Input: part model. Units: mm. Frame: model coordinates. A direction names the side the tool comes from. Give positions to 0.01 mm unless a question says otherwise; leave off trailing zeros. Loops run counter-clockwise (first coordinate to the right, second up) from the corner with the lowest first, then second, coordinate; pieces in that order, holes last. Notation, with made-up numbers: (66, 61) -> (95, 61) arc R22 cw to (95, 82) -> close; hole circle Ø8 at (-23.5, 61). An arc over 180 degrees is marked (long way). Use CSV: the item, a comma, the result in double quotes.
```python
from build123d import *

# Parameters (mm, degrees)
FILLET1_R = 3
FILLET2_R = 3


with BuildPart() as part:
    # Sketch2 → Revolve1 (revolve)
    with BuildSketch(Plane(origin=(0, 0, 0), x_dir=(0, 0, -1), z_dir=(1, 0, 0))):
        Polygon((0, 0), (0, 100), (33.5, 100), (33.5, 27), (31.5, 27), (31.5, 25), (33.5, 25), (33.5, 0), align=None)
    revolve(axis=Axis((0, 0, 0), (0, 1, 0)))

    # Fillet1
    fillet1_edges = [part.edges().sort_by_distance(p)[0] for p in [
        (0, 100, 33.5),
    ]]
    fillet(fillet1_edges, radius=FILLET1_R)

    # Fillet2
    fillet2_edges = [part.edges().sort_by_distance(p)[0] for p in [
        (0, 0, 33.5),
    ]]
    fillet(fillet2_edges, radius=FILLET2_R)


solid = part.part
```
1) Reachability of faces 4 (the cylindrical face through (32.703, 13.846, 7.262)), 5 (the flat face through (20, 25, 25)) from +Z, -Z, +X, -X, +Y, -Y: full face, straight path, thin tool, end or side. Return the list, or none.
From the geometry:
face 4,"+Y, -Y"
face 5,"none"
2) Contact query for flat-ended pins moving along their axis: pin 1 (2 mm diameter, centred on y = 14, z = -10, fed in from -X); pin 2 (2 mm diameter, centred on x = 25.5, y = 87.5, fed in from -Z); pin 3 (8 mm diameter, centred on x = -18.5, y = 41, fed in from +Z). Output: stop coordinate, or through.
From the geometry:
pin 1,"stops at x = -32.27"
pin 2,"stops at z = -22.85"
pin 3,"stops at z = 30.2"
3) Mould query, pull axis Y, two halves, no side actions, for faces 1 (the cylindrical face through (32.703, 61.51, 7.262)), 2 (the flat face through (20, 27, -25)), 3 (the flat face through (0, 100, 0)). Classes: pulls with the +Y half, pulls with the -Y half, needs draft (parallel to the pull), parting line crosses it, or undercut.
From the geometry:
face 1,"needs draft"
face 2,"undercut"
face 3,"pulls with the +Y half"
4) Section query A-A (y = 17.5). Return loops of the section in (x, z).
From the geometry:
outline,"circle Ø67 at (0, 0)"
5) Ray query, line 1 (Y direction, x = 17, z = -28.5); line 2 (Y direction, x = -18.5, z = -26.5); line 3 (X direction, y = 7.5, z = 15). Return the intervals inside material, ascending.
From the geometry:
line 1,"y = 1.66 to 25, 27 to 98.34"
line 2,"y = 0.61 to 25, 27 to 99.39"
line 3,"x = -29.95 to 29.95"
